Autodesk Inventor part; units mm, degrees
ref_plane "YZ Plane" through (0, 0, 0) normal (1, 0, 0) x (0, 1, 0)
ref_plane "XZ Plane" through (0, 0, 0) normal (0, 1, 0) x (-1, 0, 0)
ref_plane "XY Plane" through (0, 0, 0) normal (0, 0, 1) x (1, 0, 0)
sketch "Sketch1" plane through (0, 0, 0) normal (0, 0, 1) x (1, 0, 0)
  line L0 (11.5, 20) -> (-11.5, 20)
  arc A0 (-11.5, 20) -> (-13.5, 18) centre (-11.5, 18) ccw
  line L1 (-13.5, 18) -> (-13.5, -18)
  arc A1 (-13.5, -18) -> (-11.5, -20) centre (-11.5, -18) ccw
  line L2 (-11.5, -20) -> (11.5, -20)
  arc A2 (11.5, -20) -> (13.5, -18) centre (11.5, -18) ccw
  line L3 (13.5, -18) -> (13.5, 18)
  arc A3 (13.5, 18) -> (11.5, 20) centre (11.5, 18) ccw
  arc A4 (-12.7, -18) -> (-11.5, -19.2) centre (-11.5, -18) ccw
  line L4 (-12.7, -18) -> (-12.7, 18)
  arc A5 (-11.5, 19.2) -> (-12.7, 18) centre (-11.5, 18) ccw
  line L5 (-11.5, 19.2) -> (11.5, 19.2)
  arc A6 (12.7, 18) -> (11.5, 19.2) centre (11.5, 18) ccw
  line L6 (12.7, 18) -> (12.7, -18)
  arc A7 (11.5, -19.2) -> (12.7, -18) centre (11.5, -18) ccw
  line L7 (11.5, -19.2) -> (-11.5, -19.2)
  point P0 (0, 0)
extrude "Extrusion1" add sketch "Sketch1" against normal blind 1 contours L4 A5 L5 A6 L6 A7 L7 A4
sketch "Sketch2" plane through (0, 0, -1) normal (0, 0, -1) x (-1, 0, 0)
  line L0 (-7.8847, 4.0217) -> (7.8847, 4.0217)
  line L1 (7.8847, 4.0217) -> (7.8847, 0)
  line L2 (7.8847, 0) -> (-7.8847, 0)
  line L3 (-7.8847, 0) -> (-7.8847, 4.0217)
  line L4 (-7.8847, 4.0217) -> (7.8847, 0) construction
  line L5 (7.8847, 4.0217) -> (-7.8847, 0) construction
  point P0 (0, 0)
  point P1 (0, 2.0108)
extrude "Extrusion2" add sketch "Sketch2" along normal blind 0.8
sketch "Sketch3" plane through (0, 0, 0) normal (0, 0, 1) x (1, 0, 0)
  circle A0 centre (0, 7.6298) radius 9.0102
  line L0 (-1.9548, 6.22) -> (1.856, 0.0434)
  line L1 (-2.6057, 4.9897) -> (0.5711, -0.1594)
  line L2 (-0.156, 12.1852) -> (-7.1126, 10.8563)
  line L3 (-0.8751, 10.8262) -> (-7.5712, 9.547)
  line L4 (1.4903, 15.2965) -> (-0.156, 12.1852)
  line L5 (-0.8751, 10.8262) -> (-5.5003, 2.085)
  arc A1 (1.4903, 15.2965) -> (-7.1126, 10.8563) centre (0, 7.6298) ccw
  line L6 (2.674, 14.968) -> (-1.9548, 6.22)
  line L7 (-2.6057, 4.9897) -> (-4.5628, 1.2911)
  arc A2 (1.856, 0.0434) -> (2.674, 14.968) centre (0, 7.6298) ccw
  arc A3 (-7.5712, 9.547) -> (-5.5003, 2.085) centre (0, 7.6298) ccw
  arc A4 (-4.5628, 1.2911) -> (0.5711, -0.1594) centre (0, 7.6298) ccw
  dimension "d16" = 1.2
  dimension "d17" = 1.2
extrude "Extrusion3" cut sketch "Sketch3" against normal blind 0.2
sketch "Sketch4" plane through (0, 0, 0) normal (0, 0, 1) x (1, 0, 0)
  line L0 (-8.3854, -4.5453) -> (2.4185, -4.5453) construction
  line L1 (2.4185, -4.5453) -> (2.4185, -8.8273) construction
  line L2 (2.4185, -8.8273) -> (-8.3854, -8.8273) construction
  line L3 (-8.3854, -8.8273) -> (-8.3854, -4.5453) construction
  line L4 (-7.9406, -12.5453) -> (-7.9406, -4.5453)
  line L5 (-7.9406, -4.5453) -> (-4.8392, -4.5453)
  spline S0 degree 2 poles (-4.8392, -4.5453) (-3.7754, -4.5453) (-2.6754, -5.4649) (-2.5071, -6.4927) knots 0 0 0 1 2 2 2
  spline S1 degree 2 poles (-2.5071, -6.4927) (-2.4651, -6.8233) (-2.453, -7.0096) (-2.453, -7.1358) knots 0 0 0 1 2 2 2
  spline S2 degree 2 poles (-2.453, -7.1358) (-2.453, -8.2478) (-3.8174, -9.4799) (-5.0496, -9.4799) knots 0 0 0 1 2 2 2
  line L6 (-5.0496, -9.4799) -> (-5.8189, -9.4799)
  line L7 (-5.8189, -9.4799) -> (-5.8189, -12.5453)
  line L8 (-5.8189, -12.5453) -> (-7.9406, -12.5453)
  spline S3 degree 2 poles (-5.3561, -7.9713) (-5.1458, -7.9713) (-4.713, -7.6347) (-4.6469, -7.3041) knots 0 0 0 1 2 2 2
  spline S4 degree 2 poles (-4.6469, -7.3041) (-4.6108, -7.1358) (-4.6108, -6.9916) knots 0 0 0 1 1 1
  spline S5 degree 2 poles (-4.6108, -6.9916) (-4.6108, -6.5648) (-5.0195, -6.066) (-5.3321, -6.066) knots 0 0 0 1 2 2 2
  line L9 (-5.3321, -6.066) -> (-5.8189, -6.066)
  line L10 (-5.8189, -6.066) -> (-5.8189, -7.9713)
  line L11 (-5.8189, -7.9713) -> (-5.3561, -7.9713)
  line L12 (-2.0203, -12.5453) -> (-2.0203, -4.5453)
  line L13 (-2.0203, -4.5453) -> (2.686, -4.5453)
  line L14 (2.686, -4.5453) -> (2.686, -6.2222)
  line L15 (2.686, -6.2222) -> (0.1014, -6.2222)
  line L16 (0.1014, -6.2222) -> (0.1014, -7.6708)
  line L17 (0.1014, -7.6708) -> (2.5357, -7.6708)
  line L18 (2.5357, -7.6708) -> (2.5357, -9.2696)
  line L19 (2.5357, -9.2696) -> (0.1014, -9.2696)
  line L20 (0.1014, -9.2696) -> (0.1014, -10.8684)
  line L21 (0.1014, -10.8684) -> (2.7761, -10.8684)
  line L22 (2.7761, -10.8684) -> (2.7761, -12.5453)
  line L23 (2.7761, -12.5453) -> (-2.0203, -12.5453)
  line L24 (3.4252, -12.5453) -> (3.4252, -4.5453)
  line L25 (3.4252, -4.5453) -> (6.5267, -4.5453)
  spline S6 degree 2 poles (6.5267, -4.5453) (7.5905, -4.5453) (8.6905, -5.4649) (8.8588, -6.4927) knots 0 0 0 1 2 2 2
  spline S7 degree 2 poles (8.8588, -6.4927) (8.9008, -6.8233) (8.9129, -7.0096) (8.9129, -7.1358) knots 0 0 0 1 2 2 2
  spline S8 degree 2 poles (8.9129, -7.1358) (8.9129, -8.2478) (7.5485, -9.4799) (6.3163, -9.4799) knots 0 0 0 1 2 2 2
  line L26 (6.3163, -9.4799) -> (5.547, -9.4799)
  line L27 (5.547, -9.4799) -> (5.547, -12.5453)
  line L28 (5.547, -12.5453) -> (3.4252, -12.5453)
  spline S9 degree 2 poles (6.0098, -7.9713) (6.2201, -7.9713) (6.6529, -7.6347) (6.719, -7.3041) knots 0 0 0 1 2 2 2
  spline S10 degree 2 poles (6.719, -7.3041) (6.7551, -7.1358) (6.7551, -6.9916) knots 0 0 0 1 1 1
  spline S11 degree 2 poles (6.7551, -6.9916) (6.7551, -6.5648) (6.3464, -6.066) (6.0338, -6.066) knots 0 0 0 1 2 2 2
  line L29 (6.0338, -6.066) -> (5.547, -6.066)
  line L30 (5.547, -6.066) -> (5.547, -7.9713)
  line L31 (5.547, -7.9713) -> (6.0098, -7.9713)
  point P0 (0, 0)
extrude "Extrusion4" cut sketch "Sketch4" against normal blind 0.2
sketch "Sketch5" plane through (0, 0, 0) normal (0, 0, 1) x (1, 0, 0)
  line L0 (12.7, -4.0701) -> (14.5, -4.0701)
  line L1 (14.5, -4.0701) -> (-14.9684, -4.0701)
  line L2 (-14.9684, -4.0701) -> (-14.9684, -23.3701)
  line L3 (-14.9684, -23.3701) -> (14.5, -23.3701)
  line L4 (14.5, -23.3701) -> (14.5, -4.0701)
  point P0 (0, 0)
extrude "Extrusion5" cut sketch "Sketch5" against normal blind 10
properties part number "LimitSwitch Con Lid"
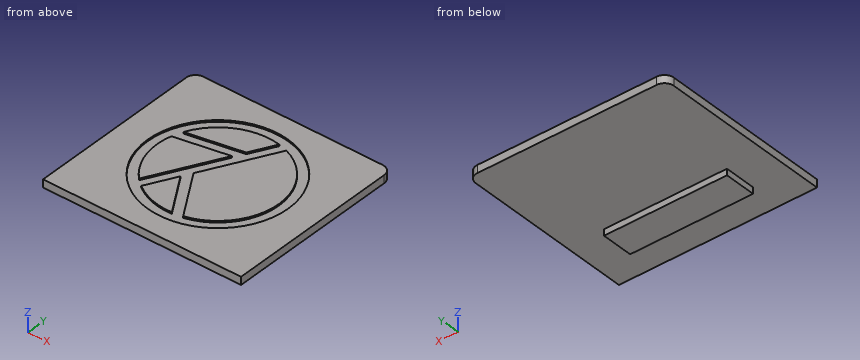
Build history of the part. All positions in model axes, mm. Coordinates: 2 decimals unless noted, no trailing zeros. Order: outer loops, then holes, each group sorted by start corner. A loop starts at its lowest first (then second) coordinate and runs counter-clockwise, first axis right, second up. Notation, with made-up numbers: M -34.75,33 L -22.75,33 A18 ccw -22.75,57 Z; hole C 81.5,41 d10. An arc over 180 degrees is marked long. One line per question, with ' | ' between items. Start each with the question number.
Q1. Saw through at C-C (y = 1). List the corners of the cut face in (x, z).
Q2. Flat gauge pins, fed straight in: pin 1 Ø0.6 at (y, z) = (2.5, -1.5) entering from +X; pin 2 Ø4 at (x, y) = (-3, 14.5) entering from +Z; pin 3 Ø0.9 at (x, z) = (1.5, -1.5) entering from -Y. Where does each tip first touch, or does it go through?
Q3. Saw through at A-A (y = 16). List the corners of the cut face in (x, z).
Q4. Probe L1, parallel to Y at x = 0, z = -0.1; L2, parallel to Y at x = -3, z = -1.3; L3, parallel to Y at x = 2, z = -0.1. List the from-to ranges inside material, lowest first. Write a range as from..to.
Q5. Saw through at D-D (x = 4.5). List the corners of the cut face in (y, z).
Q6. Saw through at B-B (x = 9.5). List the corners of the cut face in (y, z), then the cut area to 3 significant figures.
Check values:
1) outline: M -12.7,-1 L -7.88,-1 L -7.88,-1.8 L 7.88,-1.8 L 7.88,-1 L 12.7,-1 L 12.7,0 L 6.1,0 L 6.1,-0.2 L 4.13,-0.2 L 4.13,0 L 1.27,0 L 1.27,-0.2 L -0.14,-0.2 L -0.14,0 L -4.13,0 L -4.13,-0.2 L -6.1,-0.2 L -6.1,0 L -12.7,0 Z
2) pin 1: stops at x = 7.88 | pin 2: stops at z = 0 | pin 3: stops at y = 0
3) outline: M -12.7,-1 L 12.7,-1 L 12.7,0 L 3.34,0 L 3.34,-0.2 L -3.34,-0.2 L -3.34,0 L -12.7,0 Z
4) L1: y = -4.07..-1.38, -0.18..0.77, 3.05..9.91, 12.48..15.44, 16.64..19.2 | L2: y = 0..4.02 | L3: y = -4.07..-1.16, 0.08..13.69, 16.42..19.2
5) outline: M -4.07,-1 L 0,-1 L 0,-1.8 L 4.02,-1.8 L 4.02,-1 L 19.2,-1 L 19.2,0 L 15.44,0 L 15.44,-0.2 L 14.01,-0.2 L 14.01,0 L 1.25,0 L 1.25,-0.2 L -0.18,-0.2 L -0.18,0 L -4.07,0 Z
6) outline: M -4.07,-1 L 19.2,-1 L 19.2,0 L -4.07,0 Z | area: 23.3 mm2
